from build123d import *

# Parameters (mm, degrees)
SKETCH1_W           = 85
SKETCH1_H           = 30
BOSS_EXTRUDE1_DEPTH = 30
CUT_EXTRUDE1_DEPTH  = 30
SKETCH3_W           = 10
SKETCH3_H           = 10
CUT_EXTRUDE2_DEPTH  = 20
SKETCH4_R           = 2.5
CUT_EXTRUDE3_DEPTH  = 4
CUT_EXTRUDE4_START  = -3
SKETCH5_R           = 2.5
CUT_EXTRUDE4_DEPTH  = 3
SKETCH6_R           = 1
CUT_EXTRUDE5_DEPTH  = 50.348252249


with BuildPart() as part:
    # Sketch1 → Boss-Extrude1 (new body)
    with BuildSketch(Plane.XY):
        Rectangle(SKETCH1_W, SKETCH1_H)
    extrude(amount=BOSS_EXTRUDE1_DEPTH)

    # Sketch2 → Cut-Extrude1 (cut)
    with BuildSketch(Plane.XY.offset(30)):
        Polygon((-42.5, 0), (-32.5, 0), (-32.5, -4), (42.5, -4), (42.5, 15), (-42.5, 15), align=None)
        Polygon((-42.5, -10), (-32.5, -10), (-32.5, -6), (42.5, -6), (42.5, -15), (-42.5, -15), align=None)
    extrude(amount=-CUT_EXTRUDE1_DEPTH, mode=Mode.SUBTRACT)

    # Sketch3 → Cut-Extrude2 (cut)
    with BuildSketch(Plane.XY.offset(30)):
        with Locations((-37.5, -5)):
            Rectangle(SKETCH3_W, SKETCH3_H)
    extrude(amount=-CUT_EXTRUDE2_DEPTH, mode=Mode.SUBTRACT)

    # Sketch4 → Cut-Extrude3 (cut)
    with BuildSketch(Plane(origin=(0, 0, 0), x_dir=(-1, 0, 0), z_dir=(0, 0, -1))):
        with Locations((37.5, -5)):
            Circle(SKETCH4_R)
    extrude(amount=-CUT_EXTRUDE3_DEPTH, mode=Mode.SUBTRACT)

    # Sketch5 → Cut-Extrude4 (cut)
    with BuildSketch(Plane.XY.offset(10).offset(CUT_EXTRUDE4_START)):
        with Locations(Location((-37.5, -5, 0), (0, 0, 180))):
            Circle(SKETCH5_R)
    extrude(amount=CUT_EXTRUDE4_DEPTH, mode=Mode.SUBTRACT)

    # Sketch6 → Cut-Extrude5 (cut, through all)
    with BuildSketch(Plane.XY.offset(7)):
        with Locations((-37.5, -5)):
            Circle(SKETCH6_R)
    extrude(amount=-CUT_EXTRUDE5_DEPTH, mode=Mode.SUBTRACT)


solid = part.part
The model under review builds one solid part; all positions refer to its coordinate system, in mm. A direction names the side the tool comes from. Round coordinates to 2 decimals unless told otherwise and drop trailing zeros. Order: outer loops, then holes, each group sorted by start corner. A loop starts at its lowest first (then second) coordinate and runs counter-clockwise, first axis right, second up. Notation, with made-up numbers: (-30.75, 23.5) -> (2.25, 23.5) arc R22 cw to (2.25, 61.5) -> close; hole circle Ø2 at (22, -6). An arc over 180 degrees is marked (long way). Return JSON: item names as keys, results as strings.
1. The part is to be moulded in two halves that separate along Y. For faces 6 (the face through (4, -4, 15)), 7 (the face through (-39.81, -5.96, 1.97)), 8 (the face through (42.5, -5, 15)), 9 (the face through (-39.81, -4.04, 8.48)), say which applies: +Y half, -Y half, draft (parallel to the pull), parting line (faces both ways), or undercut.
Answer block:
{"face 6": "+Y half", "face 7": "undercut", "face 8": "draft", "face 9": "undercut"}
2. Take a section at D-D (x = 22.5). Write out the cut boundary in (y, z), then the cut area to 3 significant figures.
Answer block:
{"outline": "(-6, 0) -> (-4, 0) -> (-4, 30) -> (-6, 30) -> close", "area": "60.0 mm²"}
3. Take a section at C-C (z = 13.75). Write out the cut boundary in (x, y).
Answer block:
{"outline": "(-32.5, -6) -> (42.5, -6) -> (42.5, -4) -> (-32.5, -4) -> close"}
4. Insertion check: P1, Ø4, axis at x = 16.5, z = 6, coming from the -Y side; P2, Ø2, axis at y = -2.5, z = 4, coming from the +X side; P3, Ø3, axis at x = -37.5, y = -5, coming from the +Z side. Each pin has a flat end and moves straight along its axis. Give the tip position at first contact, or say it passes through.
Answer block:
{"P1": "stops at y = -6", "P2": "stops at x = -32.5", "P3": "stops at z = 7"}
5. For L1, parallel to X at y = -5, z = 9; L2, parallel to Y at x = -37.5, z = 6.15; L3, parallel to Y at x = -37.5, z = 9, list the stretches that pass through material, from the lowest coordinate up. Write a range as [from, to].
Answer block:
{"L1": "x = [-42.5, -40], [-35, 42.5]", "L2": "y = [-10, -6], [-4, 0]", "L3": "y = [-10, -7.5], [-2.5, 0]"}
6. For faces 1 (the face through (-39, -5, 7)), 2 (the face through (-32.5, -2, 5)), 3 (the face through (4, -6, 15)), 4 (the face through (-39, -5, 4)), 5 (the face through (-32.5, -5, 20)), list the 3-axis set-ups (+Z, -Z, +X, -X, +Y, -Y) from which the entire face can be reached by the end or side of a thin tool; tool diameter is ignored.
Answer block:
{"face 1": "+Z", "face 2": "+Z, -Z, +X, +Y", "face 3": "+Z, -Z, +X, -Y", "face 4": "-Z", "face 5": "+Z, -X, +Y, -Y"}
7. Take a section at A-A (y = -5). Write out the cut boundary in (x, z), then the cut area to 3 significant figures.
Answer block:
{"outline": "(-42.5, 0) -> (-40, 0) -> (-40, 4) -> (-38.5, 4) -> (-38.5, 7) -> (-40, 7) -> (-40, 10) -> (-42.5, 10) -> close; (-36.5, 4) -> (-35, 4) -> (-35, 0) -> (42.5, 0) -> (42.5, 30) -> (-32.5, 30) -> (-32.5, 10) -> (-35, 10) -> (-35, 7) -> (-36.5, 7) -> close", "area": "2,310 mm²"}
8. Take a section at B-B (x = -37.5). Write out the cut boundary in (y, z).
Answer block:
{"outline": "(-10, 0) -> (-7.5, 0) -> (-7.5, 4) -> (-6, 4) -> (-6, 7) -> (-7.5, 7) -> (-7.5, 10) -> (-10, 10) -> close; (-4, 4) -> (-2.5, 4) -> (-2.5, 0) -> (0, 0) -> (0, 10) -> (-2.5, 10) -> (-2.5, 7) -> (-4, 7) -> close"}
